from build123d import *

# Parameters (mm, degrees)
ESBO_O5_R                = 3.9
RESSALTO_EXTRUS_O2_DEPTH = 3
CORTE_EXTRUS_O3_DEPTH    = 2
FILETE1_R                = 0.5
ESBO_O8_R                = 1.925
RESSALTO_EXTRUS_O3_DEPTH = 35


with BuildPart() as part:
    # Esboço5 → Ressalto-extrusão2 (new body)
    with BuildSketch(Plane.XY):
        Circle(ESBO_O5_R)
    extrude(amount=RESSALTO_EXTRUS_O2_DEPTH)

    # Esboço7 → Corte-extrusão3 (cut)
    with BuildSketch(Plane.XY.offset(3)):
        Polygon((-0.5, -0.5), (-2.25, -0.5), (-2.25, 0.5), (-0.5, 0.5), (-0.5, 2.25), (0.5, 2.25), (0.5, 0.5), (2.25, 0.5), (2.25, -0.5), (0.5, -0.5), (0.5, -2.25), (-0.5, -2.25), align=None)
    extrude(amount=-CORTE_EXTRUS_O3_DEPTH, mode=Mode.SUBTRACT)

    # Filete1
    filete1_edges = [part.edges().sort_by_distance(p)[0] for p in [
        (-3.9, 0, 0),
        (-3.9, 0, 3),
    ]]
    fillet(filete1_edges, radius=FILETE1_R)

    # Esboço8 → Ressalto-extrusão3 (add)
    with BuildSketch(Plane(origin=(0, 0, 0), x_dir=(-1, 0, 0), z_dir=(0, 0, -1))):
        with Locations(Location((0, 0, 0), (0, 0, 180))):
            Circle(ESBO_O8_R)
    extrude(amount=RESSALTO_EXTRUS_O3_DEPTH)


solid = part.part
Here's how the part is built. I have some questions about the finished solid (model axes, mm). A direction names the side the tool comes from. Give positions to 0.01 mm unless a question says otherwise; leave off trailing zeros. Write each loop counter-clockwise with the first axis right and the second up, starting at its lowest first coordinate (ties: lowest second). Pieces come first, ordered by that corner, then holes. Notation, with made-up numbers: (-24.75, 23.25) -> (-6.75, 23.25) arc R15 ccw to (-6.75, 47.25) -> close; hole circle Ø4 at (77, 19). An arc over 180 degrees is marked (long way). Use one line per item in the form item = value. Start each with the question number.
1. Will these pins go through, and if not, where does the flat tip stop? pin 1 Ø3 at (y, z) = (3, -28.5) entering from +X; pin 2 Ø1.9 at (y, z) = (1.5, 2) entering from -X; pin 3 Ø0.9 at (y, z) = (-2, 1.5) entering from +X.
2. On a 3-axis mill with a long thin cutter (end or side, diameter ignored), from which of +Z, -Z, +X, -X, +Y, -Y can I reach the whole of each face in a straight line? I mean faces 1 (the face through (0, 0, -35)), 2 (the face through (-0.5, -1, 2)), 3 (the face through (-0.42, 1.88, -17.26)). Say none if no direction works.
3. Thinking about a two-plate mould opening in Y: for faces 4 (the face through (1, -1, 3)), 5 (the face through (0.5, -1, 2)), 6 (the face through (-2.87, 2.64, 1.49)), which applies, +Y half, -Y half, draft (parallel to the pull), parting line (faces both ways), or undercut?
4. Imagine slicing it at A-A on y = 0. List the corners of the cut face in (x, z) for me (3 decimals), plus the area to 3 significant figures.
5. Imagine slicing it at C-C on z = -13. List the corners of the cut face in (x, y) for me (3 decimals), plus the area to 3 significant figures.
6. If I drill on L1, parallel to Z at x = 0, y = -0.5; L2, parallel to Z at x = -2.5, y = 1.75; L3, parallel to Y at x = 1, z = -19, over which ranges is the centre line in solid material (lowest first)?
Entries:
q1.pin_1 = 1.21
q1.pin_2 = -3.86
q1.pin_3 = 3.58
q2.face_1 = -Z, +X, -X, +Y, -Y
q2.face_2 = +Z
q2.face_3 = -Z
q3.face_4 = draft
q3.face_5 = undercut
q3.face_6 = parting line
q4.outline = (-3.9, 0.5) arc R0.5 ccw to (-3.4, 0) -> (-1.925, 0) -> (-1.925, -35) -> (1.925, -35) -> (1.925, 0) -> (3.4, 0) arc R0.5 ccw to (3.9, 0.5) -> (3.9, 2.5) arc R0.5 ccw to (3.4, 3) -> (2.25, 3) -> (2.25, 1) -> (-2.25, 1) -> (-2.25, 3) -> (-3.4, 3) arc R0.5 ccw to (-3.9, 2.5) -> close
q4.area = 149 mm²
q5.outline = circle Ø3.85 at (0, 0)
q5.area = 11.6 mm²
q6.L1 = -35 to 1
q6.L2 = 0 to 3
q6.L3 = -1.64 to 1.64
